Part model, mm, in its own coordinate system. Face numbers are marked on the shaded views. A direction names the side the tool comes from. Round coordinates to 2 decimals unless told otherwise and drop trailing zeros. Write each loop counter-clockwise with the first axis right and the second up, starting at its lowest first coordinate (ties: lowest second). Pieces come first, ordered by that corner, then holes.
from build123d import *

# Parameters (mm, degrees)
BOSS_EXTRU_1_DEPTH      = 14.5
ESQUISSE2_R             = 1
ENL_V_MAT_EXTRU_1_DEPTH = 9
ESQUISSE4_W             = 6
ESQUISSE4_H             = 6
ENL_V_MAT_EXTRU_2_DEPTH = 4


with BuildPart() as part:
    # Esquisse1 → Boss.-Extru.1 (new, symmetric)
    with BuildSketch(Plane.XY):
        with BuildLine():
            Line((-9, -22.5), (9, -22.5))
            ThreePointArc((9, -22.5), (11.121320344, -21.621320344), (12, -19.5))
            Line((12, -19.5), (12, 19.5))
            ThreePointArc((12, 19.5), (11.121320344, 21.621320344), (9, 22.5))
            Line((9, 22.5), (-9, 22.5))
            ThreePointArc((-9, 22.5), (-11.121320344, 21.621320344), (-12, 19.5))
            Line((-12, 19.5), (-12, -19.5))
            ThreePointArc((-12, -19.5), (-11.121320344, -21.621320344), (-9, -22.5))
        make_face()
    extrude(amount=BOSS_EXTRU_1_DEPTH, both=True)

    # Esquisse2 → Enlèv. mat.-Extru.1 (cut)
    with BuildSketch(Plane.XY.offset(14.5)):
        with Locations((9, 19.5)):
            Circle(ESQUISSE2_R)
        with Locations((-9, 19.5)):
            Circle(ESQUISSE2_R)
        with Locations((-9, 8.8)):
            Circle(ESQUISSE2_R)
        with Locations((9, 8.8)):
            Circle(ESQUISSE2_R)
        with Locations((-9, -19.5)):
            Circle(ESQUISSE2_R)
        with Locations((9, -19.5)):
            Circle(ESQUISSE2_R)
    extrude(amount=-ENL_V_MAT_EXTRU_1_DEPTH, mode=Mode.SUBTRACT)

    # Esquisse4 → Enlèv. mat.-Extru.2 (cut)
    with BuildSketch(Plane.XY.offset(14.5)):
        with Locations((-9, 19.5)):
            Rectangle(ESQUISSE4_W, ESQUISSE4_H)
        with Locations((9, 19.5)):
            Rectangle(ESQUISSE4_W, ESQUISSE4_H)
        with Locations((9, 8.8)):
            Rectangle(ESQUISSE4_W, ESQUISSE4_H)
        with Locations((-9, 8.8)):
            Rectangle(ESQUISSE4_W, ESQUISSE4_H)
        with Locations((-9, -19.5)):
            Rectangle(ESQUISSE4_W, ESQUISSE4_H)
        with Locations((9, -19.5)):
            Rectangle(ESQUISSE4_W, ESQUISSE4_H)
    extrude(amount=-ENL_V_MAT_EXTRU_2_DEPTH, mode=Mode.SUBTRACT)


solid = part.part
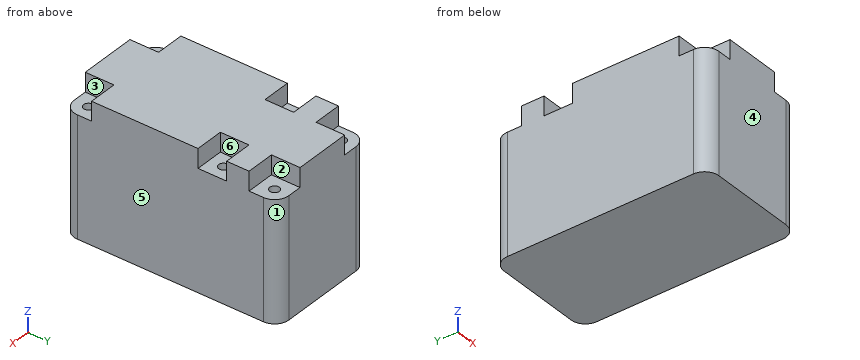
Q1. Saw through at C-C, the plane x = 6.75. Write the cut outline in (y, z), and give its area (3 significant figures).
Q2. Saw through at A-A, the plane y = 8.8. Write the cut outline in (x, z).
Q3. Two-plate mould, pull along Y, no slides. Class the marked faces 4, 5 and 6: released by +Y, released by -Y, zero draft, split by the parting line, or undercut.
Q4. Saw through at B-B, the plane x = 10.75. Write the cut outline in (y, z).
Q5. Drop flat-ended pins along their axis: P1, Ø1.6, axis at x = -9, y = -19, coming from the +Z side; P2, Ø2, axis at y = 9, z = 12.5, coming from the +X side; P3, Ø1.2, axis at x = 8.5, z = 12, coming from the -Y side. Give the stop position or say it passes through.
Q6. Wall check: line 1 (Y direction, x = -9, z = 8.95); line 2 (Z direction, x = 8, y = 18); line 3 (Z direction, x = 9.5, y = -19). Give the ranges that are in metal, low to high.
Q7. Tool access for the marked faces 1, 2 and 3: list every direction of +Z, -Z, +X, -X, +Y, -Y with a clear straight run to the whole face (end or side of a thin tool).
Computed:
1. outline: (-22.5, -14.5) - (22.5, -14.5) - (22.5, 10.5) - (16.5, 10.5) - (16.5, 14.5) - (11.8, 14.5) - (11.8, 10.5) - (5.8, 10.5) - (5.8, 14.5) - (-16.5, 14.5) - (-16.5, 10.5) - (-22.5, 10.5) - close
1. area: 1,230 mm2
2. outline: (-12, -14.5) - (12, -14.5) - (12, 10.5) - (10, 10.5) - (10, 5.5) - (8, 5.5) - (8, 10.5) - (6, 10.5) - (6, 14.5) - (-6, 14.5) - (-6, 10.5) - (-8, 10.5) - (-8, 5.5) - (-10, 5.5) - (-10, 10.5) - (-12, 10.5) - close
3. face 4: released by -Y
3. face 5: zero draft
3. face 6: undercut
4. outline: (-21.94, -14.5) - (21.94, -14.5) - (21.94, 10.5) - (16.5, 10.5) - (16.5, 14.5) - (11.8, 14.5) - (11.8, 10.5) - (5.8, 10.5) - (5.8, 14.5) - (-16.5, 14.5) - (-16.5, 10.5) - (-21.94, 10.5) - close
5. P1: stops at z = 10.5
5. P2: stops at x = 6
5. P3: stops at y = -16.5
6. line 1: y = -22.5 to -20.5, -18.5 to 7.8, 9.8 to 18.5, 20.5 to 22.5
6. line 2: z = -14.5 to 10.5
6. line 3: z = -14.5 to 5.5
7. face 1: +Z, -Z, +X, +Y
7. face 2: +Z, +X, +Y
7. face 3: +Z, +X, -Y
